Autodesk Inventor part; units mm, degrees
ref_plane "YZ Plane" through (0, 0, 0) normal (1, 0, 0) x (0, 1, 0)
ref_plane "XZ Plane" through (0, 0, 0) normal (0, 1, 0) x (-1, 0, 0)
ref_plane "XY Plane" through (0, 0, 0) normal (0, 0, 1) x (1, 0, 0)
sketch "Sketch1" plane through (0, 0, 0) normal (0, 0, 1) x (1, 0, 0)
  line L0 (-29.7166, 15.149) -> (9.9074, 15.149)
  line L1 (9.9074, 15.149) -> (9.9074, -58.765)
  line L2 (9.9074, -58.765) -> (-29.7166, -58.765)
  line L3 (-29.7166, -58.765) -> (-29.7166, 15.149)
  point P0 (0, 0)
  dimension "d0" = 39.624
  dimension "d1" = 73.914
extrude "Extrusion1" add sketch "Sketch1" along normal blind 76.2
sketch "Sketch2" plane through (0, 0, 76.2) normal (0, 0, 1) x (1, 0, 0)
  line L0 (9.9074, 15.149) -> (9.9074, -58.765)
  line L1 (-29.7166, 15.149) -> (9.9074, 15.149)
  line L2 (9.9074, 15.149) -> (9.9074, -24.475)
  line L3 (9.9074, -24.475) -> (-29.7166, -24.475)
  line L4 (-29.7166, -24.475) -> (-29.7166, 15.149)
  line L5 (-29.7166, -24.475) -> (-23.3666, -24.475)
  line L6 (-23.3666, -24.475) -> (-23.3666, -18.125)
  line L7 (-23.3666, -18.125) -> (-29.7166, -18.125)
  line L8 (-29.7166, -18.125) -> (-29.7166, -24.475)
  line L9 (-23.3666, -18.125) -> (3.5574, -18.125)
  line L10 (3.5574, -18.125) -> (3.5574, 15.149)
  line L11 (3.5574, 15.149) -> (-23.3666, 15.149)
  line L12 (-23.3666, 15.149) -> (-23.3666, -18.125)
  point P0 (0, 0)
  dimension "d4" = 39.624
  dimension "d5" = 6.35
  dimension "d6" = 6.35
  dimension "d7" = 26.924
extrude "Extrusion2" add sketch "Sketch2" along normal blind 162.56 contours L10 L9 L12 L1
sketch "Sketch3" plane through (0, 0, 238.76) normal (0, 0, 1) x (1, 0, 0)
  line L0 (-23.3666, 15.149) -> (3.5574, -18.125)
  line L1 (3.5574, 15.149) -> (-23.3666, -18.125)
  circle A0 centre (-9.9046, -1.488) radius 9.906
  point P0 (0, 0)
  dimension "d10" = 19.812
extrude "Extrusion3" cut sketch "Sketch3" against normal blind 203.2
sketch "Sketch4" plane through (0, 0, 76.2) normal (0, 0, 1) x (1, 0, 0)
  line L0 (3.5574, 15.149) -> (3.5574, -18.125)
  line L1 (3.5574, -18.125) -> (-23.3666, -18.125)
  line L2 (-23.3666, -18.125) -> (-23.3666, 15.149)
  line L3 (-29.7166, 15.149) -> (-23.3666, 15.149)
  line L4 (-29.7166, -58.765) -> (-29.7166, 15.149)
  line L5 (9.9074, -58.765) -> (-29.7166, -58.765)
  line L6 (9.9074, 15.149) -> (9.9074, -58.765)
  line L7 (3.5574, 15.149) -> (9.9074, 15.149)
  point P0 (0, 0)
extrude "Extrusion4" cut sketch "Sketch4" against normal blind 25.4
sketch "Sketch5" plane through (0, 0, 50.8) normal (0, 0, 1) x (1, 0, 0)
  line L0 (-26.5416, -21.808) -> (6.7324, -21.808)
  line L1 (6.7324, -21.808) -> (6.7324, -55.082)
  line L2 (6.7324, -55.082) -> (-26.5416, -55.082)
  line L3 (-26.5416, -55.082) -> (-26.5416, -21.808)
  point P0 (0, 0)
  dimension "d15" = 33.274
extrude "Extrusion5" add sketch "Sketch5" along normal blind 88.9
sketch "Sketch6" plane through (0, 0, 50.8) normal (0, 0, 1) x (1, 0, 0)
  line L0 (6.7324, -21.808) -> (6.7324, -55.082)
  line L1 (6.7324, -55.082) -> (-26.5416, -55.082)
  line L2 (-26.5416, -55.082) -> (-26.5416, -21.808)
  line L3 (-26.5416, -21.808) -> (6.7324, -21.808)
  line L4 (3.5574, -18.125) -> (-23.3666, -18.125)
  line L5 (-23.3666, -18.125) -> (-23.3666, 15.149)
  line L6 (-29.7166, 15.149) -> (-23.3666, 15.149)
  line L7 (-29.7166, -58.765) -> (-29.7166, 15.149)
  line L8 (9.9074, -58.765) -> (-29.7166, -58.765)
  line L9 (9.9074, 15.149) -> (9.9074, -58.765)
  line L10 (3.5574, 15.149) -> (9.9074, 15.149)
  line L11 (3.5574, 15.149) -> (3.5574, -18.125)
  point P0 (0, 0)
extrude "Extrusion6" add sketch "Sketch6" along normal blind 25.4
sketch "Sketch7" plane through (0, 0, 0) normal (0, 0, -1) x (-1, 0, 0)
  line L0 (-9.9074, 15.149) -> (-9.9074, -58.765)
  line L1 (29.7166, -58.765) -> (29.7166, 15.149)
  line L2 (-9.9074, 15.149) -> (29.7166, -24.475)
  line L3 (-9.9074, 15.149) -> (46.1294, 15.149) construction
  line L4 (29.7166, 15.149) -> (-9.9074, -24.475)
  line L5 (1.0146, 4.227) -> (18.7946, 4.227)
  line L6 (1.0146, 4.227) -> (18.7946, 4.227)
  line L7 (18.7946, 4.227) -> (18.7946, -13.553)
  line L8 (18.7946, -13.553) -> (1.0146, -13.553)
  line L9 (1.0146, -13.553) -> (1.0146, 4.227)
  point P0 (0, 0)
  dimension "d20" = 45
  dimension "d21" = 17.78
extrude "Extrusion7" add sketch "Sketch7" along normal blind 12.7 contours L5 L4 L2 | L2 L4 L9 | L4 L2 L8 | L4 L7 L2
sketch "Sketch8" plane through (-18.7946, -13.553, 0) normal (-1, 0, 0) x (0, 0, 1)
  line L0 (-12.7, 17.78) -> (-12.7, 0)
  circle A0 centre (-12.7, 8.89) radius 3.175
  point P0 (0, 13.553)
  dimension "d24" = 6.35
extrude "Extrusion8" cut sketch "Sketch8" against normal blind 25.4
sketch "Sketch9" plane through (-1.0146, -13.553, 0) normal (1, 0, 0) x (0, 0, -1)
  arc A0 (12.7, 12.065) -> (12.7, 5.715) centre (12.7, 8.89) ccw
  circle A1 centre (12.7, 8.89) radius 3.175
  circle A2 centre (12.7, 8.89) radius 8.89
  point P0 (0, 13.553)
extrude "Extrusion9" add sketch "Sketch9" against normal blind 17.78
sketch "Sketch10" plane through (0, 0, 76.2) normal (0, 0, 1) x (1, 0, 0)
  line L0 (-26.5416, -55.082) -> (6.7324, -55.082)
  line L1 (-26.5416, -21.808) -> (-26.5416, -55.082)
  line L2 (6.7324, -21.808) -> (-26.5416, -21.808)
  line L3 (6.7324, -55.082) -> (6.7324, -21.808)
  line L4 (3.5574, -18.125) -> (3.5574, 15.149)
  line L5 (-23.3666, -18.125) -> (3.5574, -18.125)
  line L6 (-23.3666, 15.149) -> (-23.3666, -18.125)
  line L7 (-29.7166, 15.149) -> (-23.3666, 15.149)
  line L8 (-29.7166, -58.765) -> (-29.7166, 15.149)
  line L9 (9.9074, -58.765) -> (-29.7166, -58.765)
  line L10 (9.9074, 15.149) -> (9.9074, -58.765)
  line L11 (3.5574, 15.149) -> (9.9074, 15.149)
  point P0 (0, 0)
extrude "Extrusion10" add sketch "Sketch10" along normal blind 38.1
fillet "Fillet1" radius 6.35 11 edges at (9.9074, 15.149, 57.15) (-29.7166, 15.149, 57.15) (9.9074, -58.765, 57.15) (-29.7166, -58.765, 57.15) (-26.5416, -55.082, 127) (6.7324, -55.082, 127) (-9.9046, -58.765, 0) (-23.3666, 15.149, 176.53) (3.5574, 15.149, 176.53) (-23.3666, -18.125, 176.53) (3.5574, -18.125, 176.53)
sketch "Sketch11" plane through (0, 0, 238.76) normal (0, 0, 1) x (1, 0, 0)
  line L0 (-17.0166, 15.149) -> (-2.7926, 15.149)
  line L1 (-2.7926, -18.125) -> (-17.0166, -18.125)
  line L2 (-9.9046, 15.149) -> (-9.9046, -4.663)
  circle A0 centre (-9.9046, -4.663) radius 9.9046
  point P0 (0, 0)
  dimension "d32" = 19.812
extrude "Extrusion11" cut sketch "Sketch11" against normal blind 101.6
sketch "Sketch12" plane through (0, 0, 238.76) normal (0, 0, 1) x (1, 0, 0)
  arc A0 (-19.6818, -3.0799) -> (-0.1273, -3.0799) centre (-9.9046, -4.663) ccw
  arc A1 (-0.1273, -3.0799) -> (-19.6818, -3.0799) centre (-9.9046, -1.488) ccw
  circle A2 centre (-9.9046, -1.488) radius 9.906
  circle A3 centre (-9.9046, -4.663) radius 9.9046
  point P0 (0, 0)
extrude "Extrusion12" add sketch "Sketch12" against normal blind 228.6 contours A3 A2 | A1 A3
sketch "Sketch13" plane through (0, 0, 238.76) normal (0, 0, 1) x (1, 0, 0)
  arc A0 (-19.6818, -3.0799) -> (-0.1273, -3.0799) centre (-9.9046, -4.663) ccw
  arc A1 (-19.6818, -3.0799) -> (-0.1273, -3.0799) centre (-9.9046, -1.488) ccw
  circle A2 centre (-9.9046, -4.663) radius 9.9046
  point P0 (0, 0)
extrude "Extrusion13" cut sketch "Sketch13" against normal blind 101.6 contours A2 A1
sketch "Sketch14" plane through (0, 0, 238.76) normal (0, 0, 1) x (1, 0, 0)
  circle A0 centre (-9.9046, -4.663) radius 9.9046
  arc A1 (-2.7926, -18.125) -> (3.5574, -11.775) centre (-2.7926, -11.775) ccw
  line L0 (3.5574, 8.799) -> (3.5574, -11.775)
  arc A2 (3.5574, 8.799) -> (-2.7926, 15.149) centre (-2.7926, 8.799) ccw
  line L1 (-17.0166, 15.149) -> (-2.7926, 15.149)
  arc A3 (-17.0166, 15.149) -> (-23.3666, 8.799) centre (-17.0166, 8.799) ccw
  line L2 (-23.3666, -11.775) -> (-23.3666, 8.799)
  arc A4 (-23.3666, -11.775) -> (-17.0166, -18.125) centre (-17.0166, -11.775) ccw
  line L3 (-2.7926, -18.125) -> (-17.0166, -18.125)
  point P0 (0, 0)
extrude "Extrusion14" add sketch "Sketch14" along normal blind 203.2
properties part number "linac body 12in"
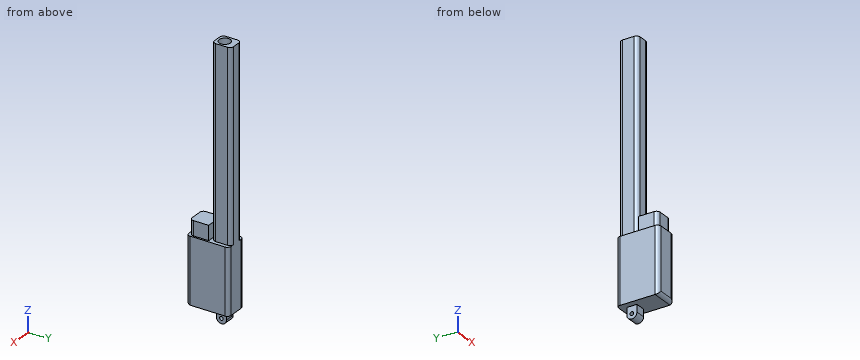
Can you work these out from the model? Positions are in its coordinate system, mm. Coordinates: 2 decimals unless noted, no trailing zeros. Order: outer loops, then holes, each group sorted by start corner. A loop starts at its lowest first (then second) coordinate and runs counter-clockwise, first axis right, second up.
1. I need wall thicknesses on line 1 (Y direction, x = -9, z = 142.5) (3 decimals); line 2 (X direction, y = -11.5, z = 240); line 3 (Z direction, x = -26.5, y = -53.5). Which ranges of each line are inside material? Lowest first, please.
2. If we section it at A-A (y = -33): Please give me the cut outline in (x, z), then the cut area to 3 significant figures.
3. If we section it at B-B (x = -9.5): Please give me the cut outline in (y, z) (3 decimals).
4. I'm going to push flat-ended pins straight in: pin 1 (12 mm diameter, centred on x = -13, y = -28, fed in from -Z); pin 2 (10 mm diameter, centred on y = -4.663, z = -12.7, fed in from +X); pin 3 (4 mm diameter, centred on x = -9, z = -4, fed in from +Y). Where does each tip first touch, or does it pass through?
Entries:
1. line 1: y = -18.125 to -14.526, 5.2 to 15.149
1. line 2: x = -23.37 to -17.07, -2.74 to 3.56
1. line 3: z = 0.09 to 114.3
2. outline: (-29.72, 0) - (9.91, 0) - (9.91, 114.3) - (6.73, 114.3) - (6.73, 139.7) - (-26.54, 139.7) - (-26.54, 114.3) - (-29.72, 114.3) - close
2. area: 5,370 mm2
3. outline: (-58.765, 6.35) arc R6.35 ccw to (-52.415, 0) - (-13.553, 0) - (-13.553, -12.7) arc R8.89 ccw to (4.227, -12.7) - (4.227, 0) - (15.149, 0) - (15.149, 441.96) - (5.233, 441.96) - (5.233, 137.16) - (-14.559, 137.16) - (-14.559, 441.96) - (-18.125, 441.96) - (-18.125, 114.3) - (-21.808, 114.3) - (-21.808, 139.7) - (-55.082, 139.7) - (-55.082, 114.3) - (-58.765, 114.3) - close; hole circle Ø6.35 at (-4.663, -12.7)
4. pin 1: stops at z = 0
4. pin 2: stops at x = -1.01
4. pin 3: stops at y = 4.23
